Can you work these out from the model? Positions are in its coordinate system, mm. Face numbers are marked on the shaded views. A direction names the side the tool comes from. Give positions to 0.01 mm unless a question says otherwise; leave off trailing zeros. Loops run counter-clockwise (first coordinate to the right, second up) from the corner with the lowest first, then second, coordinate; pieces in that order, holes last. Notation, with made-up numbers: M 41.25,-17.75 L 100.25,-17.75 A25 cw 100.25,3.25 Z; hole C -16,1.25 d4. An arc over 180 degrees is marked long. Answer as a JSON object with one key per item and string values.
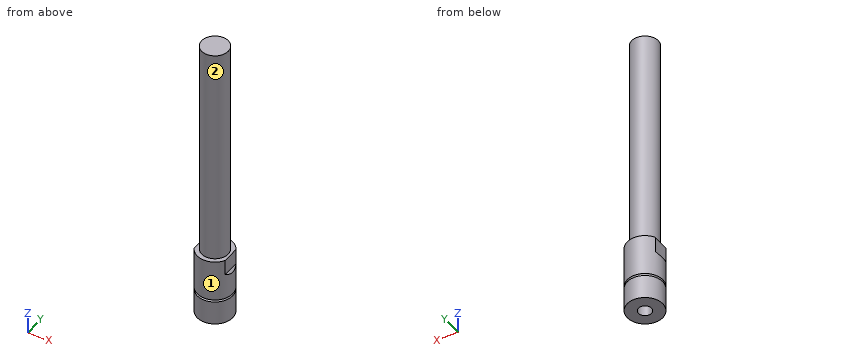
```python
from build123d import *

# Parameters (mm, degrees)
F2_W     = 19.6017324924
F2_H     = 37.1457748115
F2_W_2   = 14
F2_H_2   = 30
F3_DEPTH = 8
F4_SIZE  = 0.99999


# Not quite as in the source:
# - a fillet or chamfer is up to 0.001 mm smaller than in the source, because OpenCascade refuses the exact size


with BuildPart() as f1:
    # F0 (on Front) → F1 (revolve)
    with BuildSketch(Plane.XZ):
        with BuildLine():
            Line((2.9315422289, 21.0469197482), (2.9315422289, 0))
            Line((2.9315422289, 0), (8, 0))
            Line((8, 0), (8, 10.8380244002))
            ThreePointArc((8, 10.8380244002), (7.5, 11.3380244002), (8, 11.8380244002))
            Line((8, 11.8380244002), (8, 30.5))
            Line((8, 30.5), (6, 30.5))
            Line((6, 30.5), (6, 130.5))
            Line((6, 130.5), (0, 130.5))
            Line((0, 130.5), (0, 30.5))
            Line((0, 30.5), (0, 21.0469197482))
            Line((0, 21.0469197482), (2.9315422289, 21.0469197482))
        make_face()
    revolve(axis=Axis((0, 0, 80.5), (0, 0, 1)))

    # F2 (on face) → F3 (cut)
    with BuildSketch(Plane.XY.offset(30.5)):
        Rectangle(F2_W, F2_H)
        Rectangle(F2_W_2, F2_H_2, mode=Mode.SUBTRACT)
    extrude(amount=-F3_DEPTH, mode=Mode.SUBTRACT)

    # F4 (size 1 in the source; OpenCascade refuses exactly that, so slightly less here)
    f4_edges = [f1.edges().sort_by_distance(p)[0] for p in [
        (-7, 0, 22.5),
        (7, 0, 22.5),
    ]]
    chamfer(f4_edges, length=F4_SIZE)


solid = f1.part
```
1) Suppose I cut it at C-C, the plane z = 45.5. Write out the boundary of the cut face in (x, y), and give its area (3 significant figures).
Answer list:
{"outline": "C 0,0 d12", "area": "113 mm^2"}
2) For the marked faces 1 and 2, which set-ups out of +Z, -Z, +X, -X, +Y, -Y let a thin tool reach every point of the face, with its end or its side?
Answer list:
{"face 1": "+Z, -Z", "face 2": "+Z"}
3) Suppose I cut it at B-B, the plane z = 13. Write out the boundary of the cut face in (x, y).
Answer list:
{"outline": "C 0,0 d16; hole C 0,0 d5.86"}
4) Will these pins go through, and if not, where does the flat tip stop? pin 1 Ø6 at (y, z) = (-6, 35) entering from -X; pin 2 Ø5.5 at (y, z) = (1.5, 27.5) entering from -X; pin 3 Ø3 at (x, z) = (-0.5, 65) entering from +Y.
Answer list:
{"pin 1": "x = -5.2", "pin 2": "x = -7", "pin 3": "y = 6"}
5) Suppose I cut it at A-A, the plane x = 0. Write out the boundary of the cut face in (y, z), and give its area (3 significant figures).
Answer list:
{"outline": "M -8,0 L -2.93,0 L -2.93,21.05 L 2.93,21.05 L 2.93,0 L 8,0 L 8,10.84 A0.5 cw 8,11.84 L 8,30.5 L 6,30.5 L 6,130.5 L -6,130.5 L -6,30.5 L -8,30.5 L -8,11.84 A0.5 cw -8,10.84 Z", "area": "1,560 mm^2"}
6) Please list where these lines run through material, in increasing order: line 1 along Y through (x, z) = (0, 7.5); line 2 along Z through (x, y) = (-4.75, 5.25); line 3 along Y through (x, z) = (0, 54.5). Write a range as from..to.
Answer list:
{"line 1": "-8..-2.93, 2.93..8", "line 2": "0..30.5", "line 3": "-6..6"}
